from build123d import *

# Parameters (mm, degrees)
SKETCH_1_R          = 4
EXTRUDE_1_DEPTH     = 4
CUT_EXTRUDE_1_REACH = 127.309
SKETCH_2_R          = 1.5
EXTRUDE_2_DEPTH     = 4
FILLET_1_R          = 3
FILLET_3_R          = 10
SKETCH_4_R          = 1.5
CUT_EXTRUDE_2_DEPTH = 10


with BuildPart() as part:
    # 草图1 → 凸台-拉伸1 (new body)
    with BuildSketch(Plane(origin=(0, 0, 0), x_dir=(1, 0, 0), z_dir=(0, 1, 0))):
        with BuildLine():
            Line((100.928932188, -30.928932188), (70, 0))
            Line((70, 0), (35, 0))
            Line((35, 0), (35, 70))
            Line((35, 70), (15, 70))
            Line((15, 70), (15, 0))
            Line((15, 0), (-20, 0))
            Line((-20, 0), (-20, -20))
            Line((-20, -20), (61.715728753, -20))
            Line((61.715728753, -20), (86.786796564, -45.071067812))
            ThreePointArc((86.786796564, -45.071067812), (100.928932188, -45.071067812), (100.928932188, -30.928932188))
        make_face()
        with Locations(Location((93.857864376, -38, 0), (0, 0, 270))):
            Circle(SKETCH_1_R, mode=Mode.SUBTRACT)
    extrude(amount=EXTRUDE_1_DEPTH)

    # 草图2 → 切除-拉伸1 (cut, up to next)
    with BuildSketch(Plane(origin=(0, 4, 0), x_dir=(1, 0, 0), z_dir=(0, 1, 0)), mode=Mode.PRIVATE) as cut_extrude_1_sk1:
        with Locations(Location((17.5, 60, 0), (0, 0, 270))):
            Circle(SKETCH_2_R)
    cut_extrude_1_tool1 = extrude(cut_extrude_1_sk1.sketch, amount=-CUT_EXTRUDE_1_REACH, mode=Mode.PRIVATE) & part.part
    # 草图2 → 切除-拉伸1 (cut, up to next)
    with BuildSketch(Plane(origin=(0, 4, 0), x_dir=(1, 0, 0), z_dir=(0, 1, 0)), mode=Mode.PRIVATE) as cut_extrude_1_sk2:
        with Locations(Location((32.5, 60, 0), (0, 0, 270))):
            Circle(SKETCH_2_R)
    cut_extrude_1_tool2 = extrude(cut_extrude_1_sk2.sketch, amount=-CUT_EXTRUDE_1_REACH, mode=Mode.PRIVATE) & part.part
    # 草图2 → 切除-拉伸1 (cut, up to next)
    with BuildSketch(Plane(origin=(0, 4, 0), x_dir=(1, 0, 0), z_dir=(0, 1, 0)), mode=Mode.PRIVATE) as cut_extrude_1_sk3:
        with Locations(Location((32.5, 50, 0), (0, 0, 270))):
            Circle(SKETCH_2_R)
    cut_extrude_1_tool3 = extrude(cut_extrude_1_sk3.sketch, amount=-CUT_EXTRUDE_1_REACH, mode=Mode.PRIVATE) & part.part
    # 草图2 → 切除-拉伸1 (cut, up to next)
    with BuildSketch(Plane(origin=(0, 4, 0), x_dir=(1, 0, 0), z_dir=(0, 1, 0)), mode=Mode.PRIVATE) as cut_extrude_1_sk4:
        with Locations(Location((17.5, 50, 0), (0, 0, 270))):
            Circle(SKETCH_2_R)
    cut_extrude_1_tool4 = extrude(cut_extrude_1_sk4.sketch, amount=-CUT_EXTRUDE_1_REACH, mode=Mode.PRIVATE) & part.part
    # 草图2 → 切除-拉伸1 (cut, up to next)
    with BuildSketch(Plane(origin=(0, 4, 0), x_dir=(1, 0, 0), z_dir=(0, 1, 0)), mode=Mode.PRIVATE) as cut_extrude_1_sk5:
        with Locations(Location((17.5, 20, 0), (0, 0, 270))):
            Circle(SKETCH_2_R)
    cut_extrude_1_tool5 = extrude(cut_extrude_1_sk5.sketch, amount=-CUT_EXTRUDE_1_REACH, mode=Mode.PRIVATE) & part.part
    # 草图2 → 切除-拉伸1 (cut, up to next)
    with BuildSketch(Plane(origin=(0, 4, 0), x_dir=(1, 0, 0), z_dir=(0, 1, 0)), mode=Mode.PRIVATE) as cut_extrude_1_sk6:
        with Locations(Location((17.5, 10, 0), (0, 0, 270))):
            Circle(SKETCH_2_R)
    cut_extrude_1_tool6 = extrude(cut_extrude_1_sk6.sketch, amount=-CUT_EXTRUDE_1_REACH, mode=Mode.PRIVATE) & part.part
    # 草图2 → 切除-拉伸1 (cut, up to next)
    with BuildSketch(Plane(origin=(0, 4, 0), x_dir=(1, 0, 0), z_dir=(0, 1, 0)), mode=Mode.PRIVATE) as cut_extrude_1_sk7:
        with Locations(Location((32.5, 10, 0), (0, 0, 270))):
            Circle(SKETCH_2_R)
    cut_extrude_1_tool7 = extrude(cut_extrude_1_sk7.sketch, amount=-CUT_EXTRUDE_1_REACH, mode=Mode.PRIVATE) & part.part
    # 草图2 → 切除-拉伸1 (cut, up to next)
    with BuildSketch(Plane(origin=(0, 4, 0), x_dir=(1, 0, 0), z_dir=(0, 1, 0)), mode=Mode.PRIVATE) as cut_extrude_1_sk8:
        with Locations(Location((32.5, 20, 0), (0, 0, 270))):
            Circle(SKETCH_2_R)
    cut_extrude_1_tool8 = extrude(cut_extrude_1_sk8.sketch, amount=-CUT_EXTRUDE_1_REACH, mode=Mode.PRIVATE) & part.part
    # 草图2 → 切除-拉伸1 (cut, up to next)
    with BuildSketch(Plane(origin=(0, 4, 0), x_dir=(1, 0, 0), z_dir=(0, 1, 0)), mode=Mode.PRIVATE) as cut_extrude_1_sk9:
        with Locations(Location((42.5, -5, 0), (0, 0, 270))):
            Circle(SKETCH_2_R)
    cut_extrude_1_tool9 = extrude(cut_extrude_1_sk9.sketch, amount=-CUT_EXTRUDE_1_REACH, mode=Mode.PRIVATE) & part.part
    # 草图2 → 切除-拉伸1 (cut, up to next)
    with BuildSketch(Plane(origin=(0, 4, 0), x_dir=(1, 0, 0), z_dir=(0, 1, 0)), mode=Mode.PRIVATE) as cut_extrude_1_sk10:
        with Locations(Location((42.5, -15, 0), (0, 0, 270))):
            Circle(SKETCH_2_R)
    cut_extrude_1_tool10 = extrude(cut_extrude_1_sk10.sketch, amount=-CUT_EXTRUDE_1_REACH, mode=Mode.PRIVATE) & part.part
    # 草图2 → 切除-拉伸1 (cut, up to next)
    with BuildSketch(Plane(origin=(0, 4, 0), x_dir=(1, 0, 0), z_dir=(0, 1, 0)), mode=Mode.PRIVATE) as cut_extrude_1_sk11:
        with Locations(Location((7.5, -15, 0), (0, 0, 270))):
            Circle(SKETCH_2_R)
    cut_extrude_1_tool11 = extrude(cut_extrude_1_sk11.sketch, amount=-CUT_EXTRUDE_1_REACH, mode=Mode.PRIVATE) & part.part
    # 草图2 → 切除-拉伸1 (cut, up to next)
    with BuildSketch(Plane(origin=(0, 4, 0), x_dir=(1, 0, 0), z_dir=(0, 1, 0)), mode=Mode.PRIVATE) as cut_extrude_1_sk12:
        with Locations(Location((7.5, -5, 0), (0, 0, 270))):
            Circle(SKETCH_2_R)
    cut_extrude_1_tool12 = extrude(cut_extrude_1_sk12.sketch, amount=-CUT_EXTRUDE_1_REACH, mode=Mode.PRIVATE) & part.part
    # 草图2 → 切除-拉伸1 (cut, up to next)
    with BuildSketch(Plane(origin=(0, 4, 0), x_dir=(1, 0, 0), z_dir=(0, 1, 0)), mode=Mode.PRIVATE) as cut_extrude_1_sk13:
        with Locations(Location((60, -15, 0), (0, 0, 270))):
            Circle(SKETCH_2_R)
    cut_extrude_1_tool13 = extrude(cut_extrude_1_sk13.sketch, amount=-CUT_EXTRUDE_1_REACH, mode=Mode.PRIVATE) & part.part
    # 草图2 → 切除-拉伸1 (cut, up to next)
    with BuildSketch(Plane(origin=(0, 4, 0), x_dir=(1, 0, 0), z_dir=(0, 1, 0)), mode=Mode.PRIVATE) as cut_extrude_1_sk14:
        with Locations(Location((60, -5, 0), (0, 0, 270))):
            Circle(SKETCH_2_R)
    cut_extrude_1_tool14 = extrude(cut_extrude_1_sk14.sketch, amount=-CUT_EXTRUDE_1_REACH, mode=Mode.PRIVATE) & part.part
    # 草图2 → 切除-拉伸1 (cut, up to next)
    with BuildSketch(Plane(origin=(0, 4, 0), x_dir=(1, 0, 0), z_dir=(0, 1, 0)), mode=Mode.PRIVATE) as cut_extrude_1_sk15:
        with Locations(Location((-10, -15, 0), (0, 0, 270))):
            Circle(SKETCH_2_R)
    cut_extrude_1_tool15 = extrude(cut_extrude_1_sk15.sketch, amount=-CUT_EXTRUDE_1_REACH, mode=Mode.PRIVATE) & part.part
    # 草图2 → 切除-拉伸1 (cut, up to next)
    with BuildSketch(Plane(origin=(0, 4, 0), x_dir=(1, 0, 0), z_dir=(0, 1, 0)), mode=Mode.PRIVATE) as cut_extrude_1_sk16:
        with Locations(Location((-10, -5, 0), (0, 0, 270))):
            Circle(SKETCH_2_R)
    cut_extrude_1_tool16 = extrude(cut_extrude_1_sk16.sketch, amount=-CUT_EXTRUDE_1_REACH, mode=Mode.PRIVATE) & part.part
    add(cut_extrude_1_tool1.solids().sort_by_distance((17.5, 4, -60))[0], mode=Mode.SUBTRACT)
    add(cut_extrude_1_tool2.solids().sort_by_distance((32.5, 4, -60))[0], mode=Mode.SUBTRACT)
    add(cut_extrude_1_tool3.solids().sort_by_distance((32.5, 4, -50))[0], mode=Mode.SUBTRACT)
    add(cut_extrude_1_tool4.solids().sort_by_distance((17.5, 4, -50))[0], mode=Mode.SUBTRACT)
    add(cut_extrude_1_tool5.solids().sort_by_distance((17.5, 4, -20))[0], mode=Mode.SUBTRACT)
    add(cut_extrude_1_tool6.solids().sort_by_distance((17.5, 4, -10))[0], mode=Mode.SUBTRACT)
    add(cut_extrude_1_tool7.solids().sort_by_distance((32.5, 4, -10))[0], mode=Mode.SUBTRACT)
    add(cut_extrude_1_tool8.solids().sort_by_distance((32.5, 4, -20))[0], mode=Mode.SUBTRACT)
    add(cut_extrude_1_tool9.solids().sort_by_distance((42.5, 4, 5))[0], mode=Mode.SUBTRACT)
    add(cut_extrude_1_tool10.solids().sort_by_distance((42.5, 4, 15))[0], mode=Mode.SUBTRACT)
    add(cut_extrude_1_tool11.solids().sort_by_distance((7.5, 4, 15))[0], mode=Mode.SUBTRACT)
    add(cut_extrude_1_tool12.solids().sort_by_distance((7.5, 4, 5))[0], mode=Mode.SUBTRACT)
    add(cut_extrude_1_tool13.solids().sort_by_distance((60, 4, 15))[0], mode=Mode.SUBTRACT)
    add(cut_extrude_1_tool14.solids().sort_by_distance((60, 4, 5))[0], mode=Mode.SUBTRACT)
    add(cut_extrude_1_tool15.solids().sort_by_distance((-10, 4, 15))[0], mode=Mode.SUBTRACT)
    add(cut_extrude_1_tool16.solids().sort_by_distance((-10, 4, 5))[0], mode=Mode.SUBTRACT)

    # 草图3 → 凸台-拉伸2 (add)
    with BuildSketch(Plane(origin=(0, 4, 0), x_dir=(1, 0, 0), z_dir=(0, 1, 0))):
        Polygon((50, 0), (35, 0), (35, 20), align=None)
        Polygon((15, 0), (0, 0), (15, 20), align=None)
    extrude(amount=-EXTRUDE_2_DEPTH)

    # 圆角1
    fillet_1_edges = [part.edges().sort_by_distance(p)[0] for p in [
        (35, 2, -20),
        (50, 2, 0),
        (15, 2, -20),
        (0, 2, 0),
        (-20, 2, 20),
        (-20, 2, 0),
        (15, 2, -70),
        (35, 2, -70),
    ]]
    fillet(fillet_1_edges, radius=FILLET_1_R)

    # 圆角3
    fillet_3_edges = [part.edges().sort_by_distance(p)[0] for p in [
        (61.715728753, 2, 20),
        (70, 2, 0),
    ]]
    fillet(fillet_3_edges, radius=FILLET_3_R)

    # 草图4 → 切除-拉伸2 (cut)
    with BuildSketch(Plane(origin=(0, 4, 0), x_dir=(1, 0, 0), z_dir=(0, 1, 0))):
        with BuildLine():
            Line((-1.5, 0), (51.5, 0))
            ThreePointArc((51.5, 0), (50.158359214, 0.316718427), (49.1, 1.2))
            Line((49.1, 1.2), (35.6, 19.2))
            ThreePointArc((35.6, 19.2), (35.153950106, 20.051316702), (35, 21))
            Line((35, 21), (35, 67))
            ThreePointArc((35, 67), (34.121320344, 69.121320344), (32, 70))
            Line((32, 70), (18, 70))
            ThreePointArc((18, 70), (15.878679656, 69.121320344), (15, 67))
            Line((15, 67), (15, 21))
            ThreePointArc((15, 21), (14.846049894, 20.051316702), (14.4, 19.2))
            Line((14.4, 19.2), (0.9, 1.2))
            ThreePointArc((0.9, 1.2), (-0.158359214, 0.316718427), (-1.5, 0))
        make_face()
        with Locations((32.5, 10)):
            Circle(SKETCH_4_R, mode=Mode.SUBTRACT)
        with Locations((17.5, 20)):
            Circle(SKETCH_4_R, mode=Mode.SUBTRACT)
        with Locations((32.5, 60)):
            Circle(SKETCH_4_R, mode=Mode.SUBTRACT)
        with Locations((17.5, 50)):
            Circle(SKETCH_4_R, mode=Mode.SUBTRACT)
        with Locations((17.5, 60)):
            Circle(SKETCH_4_R, mode=Mode.SUBTRACT)
        with Locations((32.5, 50)):
            Circle(SKETCH_4_R, mode=Mode.SUBTRACT)
        with Locations((32.5, 20)):
            Circle(SKETCH_4_R, mode=Mode.SUBTRACT)
        with Locations((17.5, 10)):
            Circle(SKETCH_4_R, mode=Mode.SUBTRACT)
    extrude(amount=-CUT_EXTRUDE_2_DEPTH, mode=Mode.SUBTRACT)


solid = part.part
Can you work these out from the model? Positions are in its coordinate system, mm. Give positions to 0.01 mm unless a question says otherwise; leave off trailing zeros. Loops run counter-clockwise (first coordinate to the right, second up) from the corner with the lowest first, then second, coordinate; pieces in that order, holes last. Notation, with made-up numbers: (-40, 57) -> (6, 57) arc R27 cw to (6, 82) -> close; hole circle Ø9 at (65.5, 86). An arc over 180 degrees is marked (long way). Return JSON: item names as keys, results as strings.
Q1. I want a section at B-B, the plane z = 15. List the corners of the cut face in (x, y) for me, then the cut area to 3 significant figures.
Checks:
{"outline": "(-20, 0) -> (-11.5, 0) -> (-11.5, 4) -> (-20, 4) -> close; (-8.5, 0) -> (6, 0) -> (6, 4) -> (-8.5, 4) -> close; (9, 0) -> (41, 0) -> (41, 4) -> (9, 4) -> close; (44, 0) -> (58.5, 0) -> (58.5, 4) -> (44, 4) -> close; (61.5, 0) -> (85, 0) -> (85, 4) -> (61.5, 4) -> close", "area": "372 mm2"}
Q2. For pin 1 Ø2.5 at (x, z) = (7.5, 5) entering from +Y; pin 2 Ø1.5 at (y, z) = (0.5, 37) entering from +X; pin 3 Ø2 at (x, y) = (74.5, 0.5) entering from -Z, each with a flat end and sliding along its axis, tell me the tip position at first contact or that it passes through.
Checks:
{"pin 1": "passes through", "pin 2": "stops at x = 103.85", "pin 3": "stops at z = 3.5"}
Q3. I need wall thicknesses on probe 1 along X at (y, z) = (1.15, 16); probe 2 along X at (y, z) = (1.65, 5); probe 3 along Z at (x, y) = (43, 0.6). Which ranges of each line are inside material? Lowest first, please.
Checks:
{"probe 1": "x = -20 to -11.12, -8.88 to 6.38, 8.62 to 41.38, 43.62 to 58.88, 61.12 to 86", "probe 2": "x = -20 to -11.5, -8.5 to 6, 9 to 41, 44 to 58.5, 61.5 to 75", "probe 3": "z = 0 to 3.59, 6.41 to 13.59, 16.41 to 20"}
Q4. I want a section at C-C, the plane y = 3.05. Count the separate pieces of the cut face and the enclosed holes in it, then the cut area to 3 significant figures.
Checks:
{"separate pieces": "1", "enclosed holes": "9", "area": "2,560 mm2"}
Q5. I want a section at A-A, the plane x = 42.5. List the corners of the cut face in (y, z) for me, then the cut area to 3 significant figures.
Checks:
{"outline": "(0, 0) -> (4, 0) -> (4, 3.5) -> (0, 3.5) -> close; (0, 6.5) -> (4, 6.5) -> (4, 13.5) -> (0, 13.5) -> close; (0, 16.5) -> (4, 16.5) -> (4, 20) -> (0, 20) -> close", "area": "56.0 mm2"}
Q6. I want a section at D-D, the plane z = 38. List the corners of the cut face in (x, y) for me, then the cut area to 3 significant figures.
Checks:
{"outline": "(79.72, 0) -> (89.86, 0) -> (89.86, 4) -> (79.72, 4) -> close; (97.86, 0) -> (103.86, 0) -> (103.86, 4) -> (97.86, 4) -> close", "area": "64.6 mm2"}
Q7. We'd pull the mould along X, two halves only. Please class faces 1 (the face through (20, 2, 20)), 2 (the face through (-20, 2, 10)), 3 (the face through (41, 2, 15)): released by +X, released by -X, zero draft, split by the parting line, or undercut.
Checks:
{"face 1": "zero draft", "face 2": "released by -X", "face 3": "undercut"}
